from build123d import *

# Parameters (mm, degrees)
HOLE_WIZARD_1_D     = 4.2
HOLE_WIZARD_1_DEPTH = 4.8
HOLE_WIZARD_1_TIP   = 1.2618073
CHAMFER_1_SIZE      = 0.2
CHAMFER_2_SIZE      = 0.5


with BuildPart() as part:
    # Эскиз1 → Повернуть1 (revolve)
    with BuildSketch(Plane(origin=(0, 0, 0), x_dir=(0, 0, -1), z_dir=(1, 0, 0)), mode=Mode.PRIVATE) as revolve_1_sk:
        Polygon((-1, 21.9), (-1, 0), (-3, 0), (-3, 5), (-1.4, 5), (-1.4, 7.1), (-3.5, 7.1), (-3.5, 17.1), (-3, 17.1), (-3, 21.9), align=None)
    revolve(revolve_1_sk.sketch.rotate(Axis((0, 0, 0), (0, 1, 0)), 180), axis=Axis((0, 0, 0), (0, 1, 0)))

    # Отверстие1
    with Locations(Plane(origin=(0, 21.9, 0), x_dir=(-1, 0, 0), z_dir=(0, 1, 0))):
        with Locations((0, 0)):
            Hole(HOLE_WIZARD_1_D / 2, depth=HOLE_WIZARD_1_DEPTH)
            with Locations((0, 0, -(HOLE_WIZARD_1_DEPTH + HOLE_WIZARD_1_TIP / 2))):  # 118° drill point
                Cone(0, HOLE_WIZARD_1_D / 2, HOLE_WIZARD_1_TIP, mode=Mode.SUBTRACT)

    # Фаска1
    chamfer_1_edges = [part.edges().sort_by_distance(p)[0] for p in [
        (0, 0, 3),
        (0, 21.9, 3),
    ]]
    chamfer(chamfer_1_edges, length=CHAMFER_1_SIZE)

    # Фаска2
    chamfer_2_edges = [part.edges().sort_by_distance(p)[0] for p in [
        (0, 17.1, 3.5),
        (0, 7.1, 3.5),
    ]]
    chamfer(chamfer_2_edges, length=CHAMFER_2_SIZE - 0.0001)  # a hair under: the kernel refuses the full size


solid = part.part
Can you work these out from the model? Positions are in its coordinate system, mm. A direction names the side the tool comes from. Give positions to 0.01 mm unless a question says otherwise; leave off trailing zeros. Order: outer loops, then holes, each group sorted by start corner. A loop starts at its lowest first (then second) coordinate and runs counter-clockwise, first axis right, second up. Notation, with made-up numbers: M 30.5,0.5 L 55.5,0.5 A17 cw 55.5,5.5 Z; hole C 89,-32.75 d5. An arc over 180 degrees is marked long. Use one line per item in the form item = value.
Item 1: Thinking about a two-plate mould opening in Z: for faces 1 (the cylindrical face through (-0.9, 19.43, -2.86)), 2 (the cylindrical face through (1, 8, 0)), 3 (the flat face through (0, 0, 1.2)), which applies, pulls with the +Z half, pulls with the -Z half, needs draft (parallel to the pull), parting line crosses it, or undercut?
Values follow:
face_1 = parting line crosses it
face_2 = undercut
face_3 = needs draft
Item 2: For faces 4 (the cylindrical face through (1.341, 12.163, -3.233)), 5 (the cylindrical face through (-0.9, 2.63, -2.86)), 6 (the cylindrical face through (2.003, 19.466, 0.631)), 7 (the cylindrical face through (-0.06, 6.06, 1.4)), which set-ups out of +Z, -Z, +X, -X, +Y, -Y let a thin tool reach every point of the face, with its end or its side?
Values follow:
face_4 = +Y, -Y
face_5 = -Y
face_6 = +Y
face_7 = none
Item 3: Will these pins go through, and if not, where does the flat tip stop? pin 1 Ø1 at (y, z) = (3, 0) entering from -X; pin 2 Ø1 at (x, z) = (2.5, -2) entering from +Y; pin 3 Ø2.5 at (x, z) = (0, 0) entering from +Y; pin 4 Ø1.8 at (x, z) = (0, 0.5) entering from +Y.
Values follow:
pin_1 = -3
pin_2 = 21.9
pin_3 = 16.59
pin_4 = 16.68
Item 4: If we section it at D-D, the plane y = 6.25: Write out the boundary of the cut face in (x, z).
Values follow:
outline = C 0,0 d2.8; hole C 0,0 d2
Item 5: If I drill on line 1 along X through (y, z) = (20.4, 0); line 2 along X through (y, z) = (11.75, 0); line 3 along Y through (x, z) = (1.5, 2), over which ranges is the centre line in solid material (lowest first)? Write a range as [from, to].
Values follow:
line_1 = [-3, -2.1], [2.1, 3]
line_2 = [-3.5, -1], [1, 3.5]
line_3 = [0, 5], [7.1, 21.9]
Item 6: If we section it at C-C, the plane y = 18.5: Write out the boundary of the cut face in (x, z), and give its area (3 significant figures).
Values follow:
outline = C 0,0 d6; hole C 0,0 d4.2
area = 14.4 mm^2
